The model under review builds one solid part; all positions refer to its coordinate system, in mm. Face numbers are marked on the shaded views. A direction names the side the tool comes from. Give positions to 0.01 mm unless a question says otherwise; leave off trailing zeros. Write each loop counter-clockwise with the first axis right and the second up, starting at its lowest first coordinate (ties: lowest second). Pieces come first, ordered by that corner, then holes.
from build123d import *

# Parameters (mm, degrees)
M3_TAPPED_HOLE1_D     = 2.5
M3_TAPPED_HOLE1_DEPTH = 2
M3_TAPPED_HOLE1_TIP   = 0.751075774
CUT_EXTRUDE1_START    = -10
CUT_EXTRUDE1_DEPTH    = 10


with BuildPart() as part:
    # Sketch1 → Revolve1 (revolve)
    with BuildSketch(Plane.XY):
        with BuildLine():
            Line((0, 0), (0, 2))
            Line((0, 2), (12, 2))
            Line((12, 2), (12, 3.5))
            Line((12, 3.5), (14, 3.5))
            Line((14, 3.5), (14, 13.75))
            Line((14, 13.75), (40.5, 13.75))
            Line((40.5, 13.75), (40.5, 12.75))
            ThreePointArc((40.5, 12.75), (40.792893219, 13.457106781), (41.5, 13.75))
            Line((41.5, 13.75), (78, 13.75))
            Line((78, 13.75), (78, 0))
            Line((78, 0), (0, 0))
        make_face()
    revolve(axis=Axis((78, 0, 0), (-1, 0, 0)))

    # M3 Tapped Hole1
    with Locations(Plane(origin=(14, 0, -10), x_dir=(0, -1, 0), z_dir=(-1, 0, 0))):
        with Locations((0, 0), (0, 20)):
            Hole(M3_TAPPED_HOLE1_D / 2, depth=M3_TAPPED_HOLE1_DEPTH)
            with Locations((0, 0, -(M3_TAPPED_HOLE1_DEPTH + M3_TAPPED_HOLE1_TIP / 2))):  # 118° drill point
                Cone(0, M3_TAPPED_HOLE1_D / 2, M3_TAPPED_HOLE1_TIP, mode=Mode.SUBTRACT)

    # Sketch4 → Cut-Extrude1 (cut)
    with BuildSketch(Plane.ZY.offset(CUT_EXTRUDE1_START)):
        with BuildLine():
            Line((-1.322875656, 1.5), (1.322875656, 1.5))
            ThreePointArc((1.322875656, 1.5), (0, 2), (-1.322875656, 1.5))
        make_face()
    extrude(amount=CUT_EXTRUDE1_DEPTH, mode=Mode.SUBTRACT)


solid = part.part
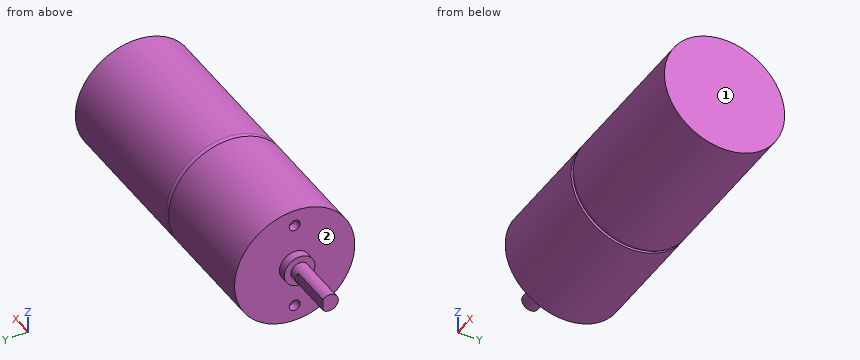
1) Consider section A-A, the plane z = 0. Give the boundary of the cut face in (x, y), then the cut area to 3 significant figures.
2) Insertion check: pin 1 (12 mm diameter, centred on y = 2.5, z = 9.5, fed in from -X); pin 2 (1.3 mm diameter, centred on x = 3.5, z = 0, fed in from +Y); pin 3 (2 mm diameter, centred on x = 60.5, z = 7, fed in from -Y). Each pin has a flat end and moves straight along its axis. Give the tip position at first contact, or say it passes through.
3) Tool access review of the marked faces 1 and 2: name each direction out of +Z, -Z, +X, -X, +Y, -Y from which nothing blocks a thin tool from reaching the whole face with its end or side.
4) To check wall thickness, follow probe 1 along Z at (x, y) = (15.15, 0); probe 2 along X at (y, z) = (10.5, 1.5); probe 3 along Y at (x, z) = (15.3, -10). State the ranges of each line that lie inside material, in increasing order.
5) Consider section B-B, the plane x = 72. Give the boundary of the cut face in (y, z), then the cut area to 3 significant figures.
Answer block:
1. outline: (0, -2) - (12, -2) - (12, -3.5) - (14, -3.5) - (14, -13.75) - (40.5, -13.75) - (40.5, -12.75) arc R1 ccw to (41.5, -13.75) - (78, -13.75) - (78, 13.75) - (41.5, 13.75) arc R1 ccw to (40.5, 12.75) - (40.5, 13.75) - (14, 13.75) - (14, 3.5) - (12, 3.5) - (12, 2) - (10, 2) - (10, 1.5) - (0, 1.5) - close
1. area: 1,820 mm2
2. pin 1: stops at x = 14
2. pin 2: stops at y = 1.5
2. pin 3: stops at y = -12.37
3. face 1: +Z, -Z, +X, +Y, -Y
3. face 2: -X
4. probe 1: z = -13.75 to -11.25, -8.75 to 8.75, 11.25 to 13.75
4. probe 2: x = 14 to 78
4. probe 3: y = -9.44 to -1.25, 1.25 to 9.44
5. outline: circle Ø27.5 at (0, 0)
5. area: 594 mm2
